Part model, mm, in its own coordinate system. Give positions to 0.01 mm unless a question says otherwise; leave off trailing zeros. Write each loop counter-clockwise with the first axis right and the second up, starting at its lowest first coordinate (ties: lowest second). Pieces come first, ordered by that corner, then holes. Notation, with made-up numbers: M -36.75,-32 L 18.25,-32 A25 ccw 18.25,-6 Z; hole C 30.5,64.5 d6. An arc over 180 degrees is marked long. Use CSV: the item, a comma, the result in double quotes. Start each with the question number.
1. Drop a flat-ended pin along its axis: pin 1 Ø1.5 at (y, z) = (69.5, 5.5) entering from -X. Give the stop position or say it passes through.
2. Band-saw the part on B-B, the plane z = 8.5. List the corners of the cut face in (x, y) (1 decimal), then the cut area to 3 significant figures.
3. Band-saw the part on C-C, the plane x = 593. List the corners of the cut face in (y, z).
4. Band-saw the part on A-A, the plane y = 72. List the corners of the cut face in (x, z), then the cut area to 3 significant figures.
5. Drill centre lines: line 1 along Y through (x, z) = (344, 14.75); line 2 along Y through (x, z) = (961, 7.5). Where is each one in solid material? Low to high. Write a range as from..to.
6. Band-saw the part on D-D, the plane y = 23. List the corners of the cut face in (x, z), then the cut area to 3 significant figures.
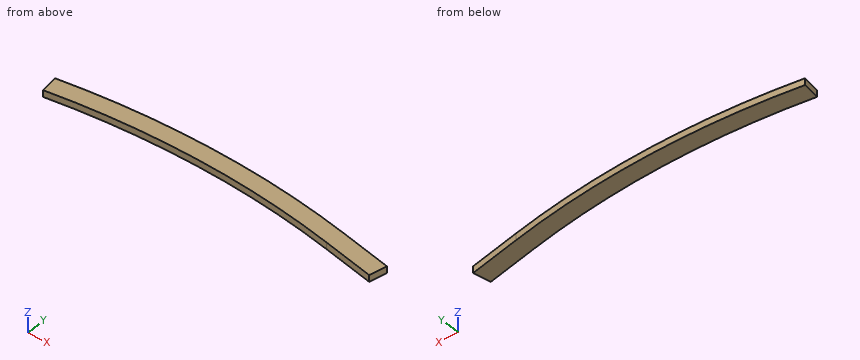
Autodesk Inventor part; units mm, degrees
ref_plane "YZ Plane" through (0, 0, 0) normal (1, 0, 0) x (0, 1, 0)
ref_plane "XZ Plane" through (0, 0, 0) normal (0, 1, 0) x (-1, 0, 0)
ref_plane "XY Plane" through (0, 0, 0) normal (0, 0, 1) x (1, 0, 0)
sketch "Sketch1" plane through (0, 0, 0) normal (0, 0, 1) x (1, 0, 0)
  line L0 (0.0002, 105.7836) -> (7.461, 55.5344)
  arc A0 (845.4951, 31.1517) -> (7.461, 55.5344) centre (358.1185, -2306.1754) ccw
  line L1 (845.4951, 31.1517) -> (994.6862, 0.0425)
  line L2 (994.6862, 0.0425) -> (1005.0559, 49.7729)
  line L3 (1005.0559, 49.7729) -> (855.8648, 80.8821)
  arc A1 (855.8648, 80.8821) -> (0.0002, 105.7836) centre (358.1185, -2306.1754) ccw
extrude "Extrusion1" add sketch "Sketch1" along normal blind 19.05
properties part number "nd-i"
Output:
1,pin 1,"stops at x = 5.28"
2,outline,"M 0,105.8 L 7.5,55.5 A2387.6 cw 845.5,31.2 L 994.7,0 L 1005.1,49.8 L 855.9,80.9 A2438.4 ccw Z"
2,area,"51,000 mm²"
3,outline,"M 69.84,0 L 120.89,0 L 120.89,19.05 L 69.84,19.05 Z"
4,outline,"M 5.02,0 L 146.19,0 L 146.19,19.05 L 5.02,19.05 Z; M 570.05,0 L 898.46,0 L 898.46,19.05 L 570.05,19.05 Z"
4,area,"8,950 mm²"
5,line 1,"y = 81.38..132.18"
5,line 2,"y = 7.07..58.96"
6,outline,"M 884.59,0 L 999.47,0 L 999.47,19.05 L 884.59,19.05 Z"
6,area,"2,190 mm²"
